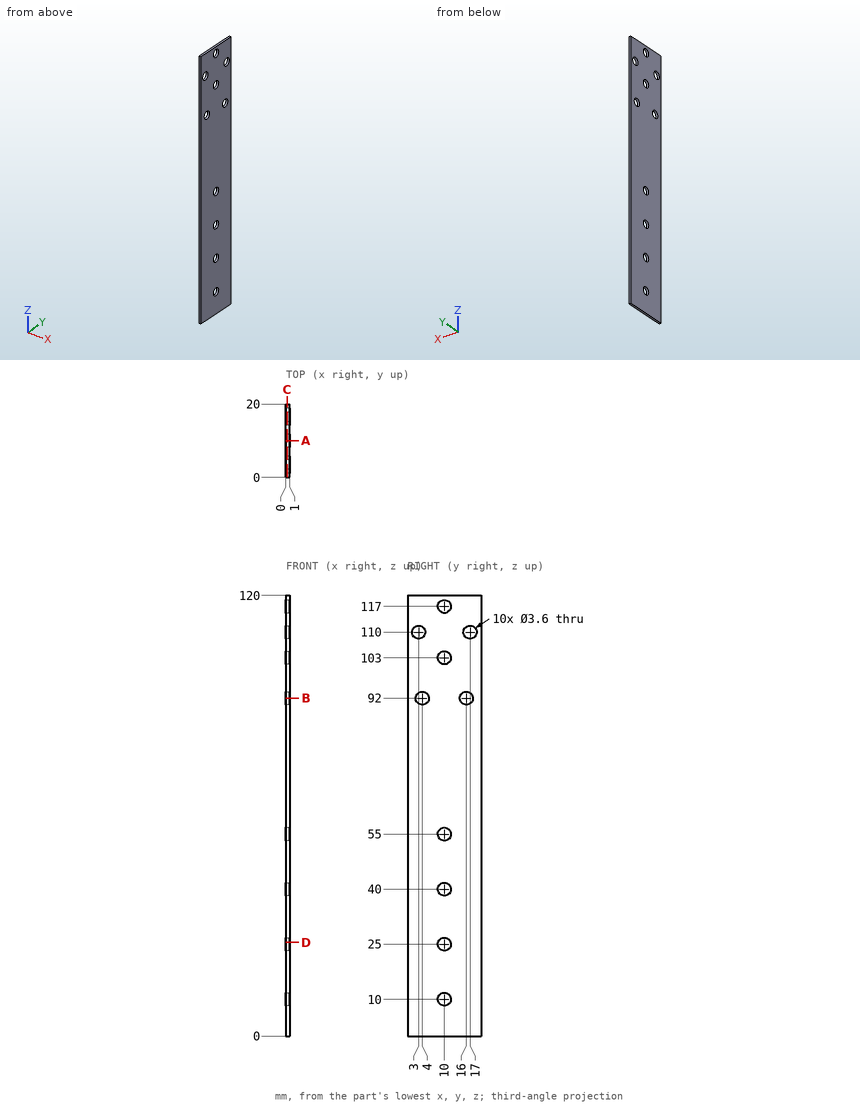
Here's the drawing with two shaded views (mm, measured from the low corner). I have some questions. Give positions to 0.01 mm unless a question says otherwise; leave off trailing zeros. Write each loop counter-clockwise with the first axis right and the second up, starting at its lowest first coordinate (ties: lowest second). Pieces come first, ordered by that corner, then holes. Notation, with made-up numbers: (19.5, 59) - (25.5, 59) arc R26 ccw to (25.5, 85) - close; hole circle Ø2 at (54, 11). An arc over 180 degrees is marked (long way). One line per item, written item: value. Start each with the question number.
Item 1: Imagine slicing it at D-D, the plane z = 25.5. List the corners of the cut face in (x, y) for me.
Item 2: Imagine slicing it at B-B, the plane z = 92. List the corners of the cut face in (x, y) for me, and give its area (3 significant figures).
Item 3: Imagine slicing it at A-A, the plane y = 10. List the corners of the cut face in (x, z) for me, and give its area (3 significant figures).
Item 4: Imagine slicing it at C-C, the plane x = 0.35. Give the number of separate pieces and of enclosed holes in the cut face, and give its area (3 significant figures).
Item 5: Please list where these lines run through material, in increasing order: line 1 (Y direction, x = 0.7, z = 92); line 2 (Y direction, x = 0.45, z = 110); line 3 (Y direction, x = 0.3, z = 117). Write a range as from..to.
Item 6: I'm going to push a flat-ended pin straight in: pin 1 (3 mm diameter, centred on y = 17, z = 110, fed in from -X). Where does the tip first touch, or does it pass through?
Geometry says:
1. outline: (0, 0) - (1, 0) - (1, 8.27) - (0, 8.27) - close; (0, 11.73) - (1, 11.73) - (1, 20) - (0, 20) - close
2. outline: (0, 0) - (1, 0) - (1, 2.2) - (0, 2.2) - close; (0, 5.8) - (1, 5.8) - (1, 14.2) - (0, 14.2) - close; (0, 17.8) - (1, 17.8) - (1, 20) - (0, 20) - close
2. area: 12.8 mm^2
3. outline: (0, 0) - (1, 0) - (1, 8.2) - (0, 8.2) - close; (0, 11.8) - (1, 11.8) - (1, 23.2) - (0, 23.2) - close; (0, 26.8) - (1, 26.8) - (1, 38.2) - (0, 38.2) - close; (0, 41.8) - (1, 41.8) - (1, 53.2) - (0, 53.2) - close; (0, 56.8) - (1, 56.8) - (1, 101.2) - (0, 101.2) - close; (0, 104.8) - (1, 104.8) - (1, 115.2) - (0, 115.2) - close; (0, 118.8) - (1, 118.8) - (1, 120) - (0, 120) - close
3. area: 98.4 mm^2
4. separate pieces: 1
4. enclosed holes: 10
4. area: 2,300 mm^2
5. line 1: 0..2.2, 5.8..14.2, 17.8..20
5. line 2: 0..1.2, 4.8..15.2, 18.8..20
5. line 3: 0..8.2, 11.8..20
6. pin 1: through
